from build123d import *

# Parameters (mm, degrees)
F1_DEPTH = 307.34
F2_R     = 63.5
F3_R     = 63.5
F4_T     = -12.7


with BuildPart() as f1:
    # F0 (on Top) → F1 (new body)
    with BuildSketch(Plane.XY):
        with BuildLine():
            Line((649.227738, 191.499934), (158.845842, 191.499934))
            Line((158.845842, 191.499934), (158.845842, -78.352302))
            Line((158.845842, -78.352302), (-197.068691, -78.352302))
            Line((-197.068691, -78.352302), (-197.068691, -377.061605))
            Line((-197.068691, -377.061605), (400.637456, -377.061605))
            ThreePointArc((400.637456, -377.061605), (473.447864, -201.281731), (649.227738, -128.471323))
            Line((649.227738, -128.471323), (649.227738, 191.499934))
        make_face()
    extrude(amount=F1_DEPTH)

    # F2
    f2_edges = [f1.edges().sort_by_distance(p)[0] for p in [
        (158.845842, 191.499934, 153.67),
        (158.845842, -78.352302, 153.67),
        (-197.068691, -78.352302, 153.67),
        (-197.068691, -377.061605, 153.67),
        (649.227738, -128.471323, 153.67),
        (400.637456, -377.061605, 153.67),
        (649.227738, 191.499934, 153.67),
    ]]
    fillet(f2_edges, radius=F2_R)

    # F3
    f3_edges = [f1.edges().sort_by_distance(p)[0] for p in [
        (473.447864, -201.281731, 307.34),
        (383.739621, -362.819492, 307.34),
        (634.985625, -111.573488, 307.34),
        (105.048558, -377.061605, 307.34),
        (649.227738, 28.25013, 307.34),
        (-178.469972, -358.462886, 307.34),
        (630.629019, 172.901214, 307.34),
        (-197.068691, -227.706954, 307.34),
        (404.03679, 191.499934, 307.34),
        (-178.469972, -96.951022, 307.34),
        (177.444561, 172.901214, 307.34),
        (-19.111425, -78.352302, 307.34),
        (158.845842, 56.573816, 307.34),
        (140.247122, -59.753583, 307.34),
    ]]
    fillet(f3_edges, radius=F3_R)

    # F4
    f4_openings = [f1.faces().sort_by_distance(p)[0] for p in [
        (250.443823, -109.892421, 0),
    ]]
    offset(amount=F4_T, openings=f4_openings)


solid = f1.part
Part model, mm, in its own coordinate system. A direction names the side the tool comes from. Give positions to 0.01 mm unless a question says otherwise; leave off trailing zeros. Loops run counter-clockwise (first coordinate to the right, second up) from the corner with the lowest first, then second, coordinate; pieces in that order, holes last. Notation, with made-up numbers: M 71,-32 L 116,-32 A18 ccw 116,-9 Z; hole C 4,-9.5 d2. An arc over 180 degrees is marked long. Put each result on its own line as item: value. Start each with the question number.
1) Pull direction Y, two halves, no side cores. Call faces 3 (the flat face through (158.846, 58, 120)), 4 (the cylindrical face through (630.133, 173.392, 123.627)), 5 (the cylindrical face through (108.39, -349.09, 280.15)): +Y half, -Y half, draft (parallel to the pull), parting line (faces both ways), or undercut.
2) Probe probe 1 along Y at (x, z) = (84, 172); probe 2 along X at (y, z) = (100.5, 93); probe 3 along Y at (x, z) = (276.5, 98). List the from-to ranges inside material, lowest first.
3) Saw through at D-D (z = 267.5). List the corners of the cut face in (x, y), then the cut area to 3 significant figures.
4) Saw through at A-A (z = 153). List the corners of the cut face in (x, y), then the cut area to 3 significant figures.
5) Saw through at C-C (y = 118). List the corners of the cut face in (x, z), then the cut area to 3 significant figures.
6) Saw through at B-B (x = -109). List the corners of the cut face in (y, z).
7) 3-axis set-ups, long thin cutter, end or side, ignore diameter. For faces 1 (the cylindrical face through (383.27, -363.2, 123.63)), 2 (the cylindrical face through (624.83, -103.93, 123.63)): which of +Z, -Z, +X, -X, +Y, -Y reach the whole face in a straight line?
8) Flat gauge pins, fed straight in: pin 1 (1.5 mm diameter, centred on x = 428, y = -8.5, fed in from -Z); pin 2 (1.5 mm diameter, centred on x = 186.5, y = -70.5, fed in from +Z); pin 3 (10 mm diameter, centred on y = -210.5, z = 164.5, fed in from +X). Where does each tip first touch, or does it go through?
Numbers:
1. face 3: draft
1. face 4: +Y half
1. face 5: undercut
2. probe 1: -377.06 to -364.36, -91.05 to -78.35
2. probe 2: 158.85 to 171.55, 636.53 to 649.23
2. probe 3: -377.06 to -364.36, 178.8 to 191.5
3. outline: M -192.5,-313.56 A58.93 ccw -133.57,-372.49 L 343.67,-372.49 A58.93 ccw 401.36,-325.55 A253.16 cw 597.72,-129.19 A58.93 ccw 644.66,-71.5 L 644.66,128 A58.93 ccw 585.73,186.93 L 222.35,186.93 A58.93 ccw 163.42,128 L 163.42,-14.85 A68.07 cw 95.35,-82.92 L -133.57,-82.92 A58.93 ccw -192.5,-141.85 Z; hole M -178.52,-313.56 A44.95 ccw -133.57,-358.52 L 343.67,-358.52 A44.95 ccw 387.68,-322.71 A267.14 cw 594.87,-115.51 A44.95 ccw 630.68,-71.5 L 630.68,128 A44.95 ccw 585.73,172.95 L 222.35,172.95 A44.95 ccw 177.39,128 L 177.39,-14.85 A82.05 cw 95.35,-96.9 L -133.57,-96.9 A44.95 ccw -178.52,-141.85 Z
3. area: 34,500 mm^2
4. outline: M -197.07,-313.56 A63.5 ccw -133.57,-377.06 L 343.67,-377.06 A63.5 ccw 405.84,-326.48 A248.59 cw 598.65,-133.67 A63.5 ccw 649.23,-71.5 L 649.23,128 A63.5 ccw 585.73,191.5 L 222.35,191.5 A63.5 ccw 158.85,128 L 158.85,-14.85 A63.5 cw 95.35,-78.35 L -133.57,-78.35 A63.5 ccw -197.07,-141.85 Z; hole M -184.37,-313.56 A50.8 ccw -133.57,-364.36 L 343.67,-364.36 A50.8 ccw 393.4,-323.9 A261.29 cw 596.06,-121.24 A50.8 ccw 636.53,-71.5 L 636.53,128 A50.8 ccw 585.73,178.8 L 222.35,178.8 A50.8 ccw 171.55,128 L 171.55,-14.85 A76.2 cw 95.35,-91.05 L -133.57,-91.05 A50.8 ccw -184.37,-141.85 Z
4. area: 31,800 mm^2
5. outline: M 158.85,0 L 171.55,0 L 171.55,243.84 A50.8 cw 222.35,294.64 L 585.73,294.64 A50.8 cw 636.53,243.84 L 636.53,0 L 649.23,0 L 649.23,243.84 A63.5 ccw 585.73,307.34 L 222.35,307.34 A63.5 ccw 158.85,243.84 Z
5. area: 13,100 mm^2
6. outline: M -377.06,0 L -364.36,0 L -364.36,243.84 A50.8 cw -313.56,294.64 L -141.85,294.64 A50.8 cw -91.05,243.84 L -91.05,0 L -78.35,0 L -78.35,243.84 A63.5 ccw -141.85,307.34 L -313.56,307.34 A63.5 ccw -377.06,243.84 Z
7. face 1: +Z, -Z, +X, -Y
7. face 2: -Z
8. pin 1: z = 294.64
8. pin 2: z = 304.29
8. pin 3: x = 469.33
